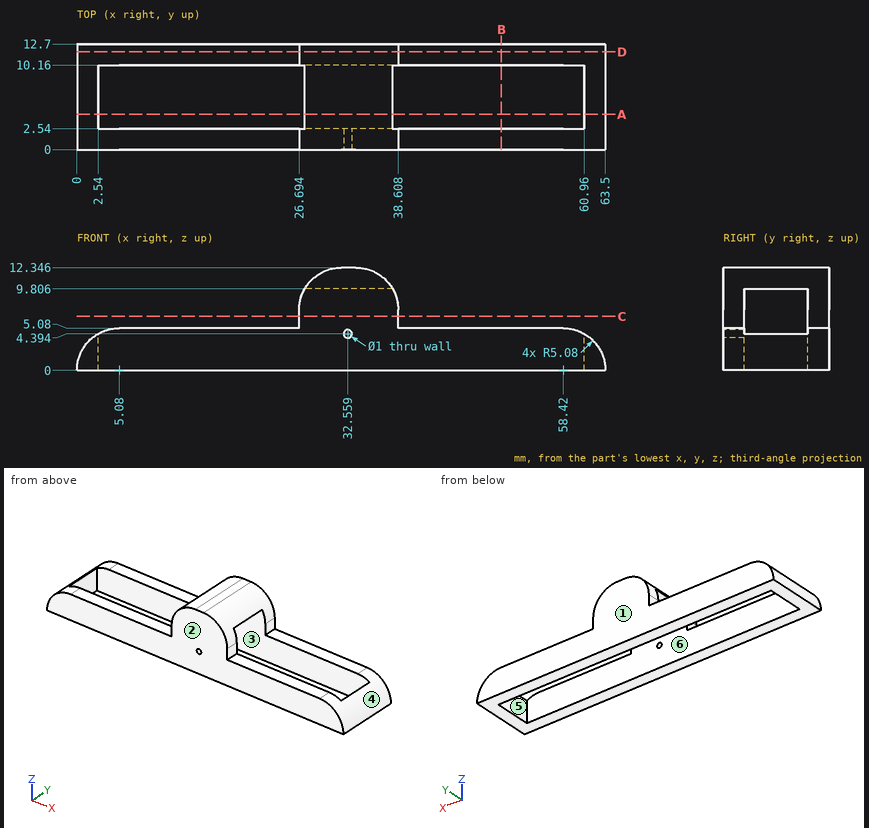
Could you check a few things on this drawing? It's one solid part, dimensions in mm from its lowest x, y, z. A direction names the side the tool comes from. Coordinates: 2 decimals unless noted, no trailing zeros. Order: outer loops, then holes, each group sorted by start corner. A loop starts at its lowest first (then second) coordinate and runs counter-clockwise, first axis right, second up. Notation, with made-up numbers: (53.25, 66.25) -> (78.25, 66.25) arc R31 ccw to (78.25, 95.25) -> close; hole circle Ø3 at (10, -14). An arc over 180 degrees is marked (long way). One line per item, written item: value. Start each with the question number.
1) Imagine slicing it at B-B on x = 51. List the corners of the cut face in (y, z) for me, plus the area to 3 significant figures.
2) Imagine slicing it at A-A on y = 4.25. List the corners of the cut face in (x, z) for me (1 decimal).
3) I'm going to push flat-ended pins straight in: pin 1 (2 mm diameter, centred on y = 6, z = 3, fed in from -X); pin 2 (1.1 mm diameter, centred on y = 11.5, z = 6.5, fed in from -X); pin 3 (6 mm diameter, centred on y = 5.5, z = 7.5, fed in from +X); pin 4 (4 mm diameter, centred on x = 53, y = 5.5, fed in from -Z). Where does each tip first touch, or does it pass through?
4) Imagine slicing it at C-C on z = 6.5. List the corners of the cut face in (x, y) for me.
5) If I drill on L1, parallel to Y at x = 49.5, z = 4.5; L2, parallel to Z at x = 17, y = 12; L3, parallel to X at y = 1.5, z = 6.5, over which ranges is the centre line in solid material (lowest first)? Write a range as [from, to].
6) Imagine slicing it at D-D on y = 11.75. List the corners of the cut face in (x, z) for me.
7) We'd pull the mould along Y, two halves only. Please class the marked faces 1, 2 and 3: +Y half, -Y half, draft (parallel to the pull), parting line (faces both ways), or undercut.
8) Which directions (+Z, -Z, +X, -X, +Y, -Y) give clear straight access to the entire face, cutting with the end or side of a thin tool? Please do the marked faces 4, 5 and 6.
Answer list:
1. outline: (0, 0) -> (2.54, 0) -> (2.54, 5.08) -> (0, 5.08) -> close; (10.16, 0) -> (12.7, 0) -> (12.7, 5.08) -> (10.16, 5.08) -> close
1. area: 25.8 mm2
2. outline: (0, 0) -> (2.5, 0) -> (2.5, 4.4) arc R5.1 ccw to start; (27.4, 9.8) -> (37.9, 9.8) arc R5.1 ccw to (33.5, 12.3) -> (31.8, 12.3) arc R5.1 ccw to start; (61, 0) -> (63.5, 0) arc R5.1 ccw to (61, 4.4) -> close
3. pin 1: stops at x = 0.41
3. pin 2: stops at x = 26.69
3. pin 3: stops at x = 38.61
3. pin 4: passes through
4. outline: (26.69, 0) -> (38.61, 0) -> (38.61, 2.54) -> (26.69, 2.54) -> close; (26.69, 10.16) -> (38.61, 10.16) -> (38.61, 12.7) -> (26.69, 12.7) -> close
5. L1: y = [0, 2.54], [10.16, 12.7]
5. L2: z = [0, 5.08]
5. L3: x = [26.69, 38.61]
6. outline: (0, 0) -> (63.5, 0) arc R5.08 ccw to (58.42, 5.08) -> (38.61, 5.08) -> (38.61, 7.27) arc R5.08 ccw to (33.53, 12.35) -> (31.77, 12.35) arc R5.08 ccw to (26.69, 7.27) -> (26.69, 5.08) -> (5.08, 5.08) arc R5.08 ccw to start
7. face 1: +Y half
7. face 2: -Y half
7. face 3: undercut
8. face 4: +Z, +X, +Y, -Y
8. face 5: +Z, -Z
8. face 6: -Z
